Build history of the part. All positions in model axes, mm. Give positions to 0.01 mm unless a question says otherwise; leave off trailing zeros. Write each loop counter-clockwise with the first axis right and the second up, starting at its lowest first coordinate (ties: lowest second). Pieces come first, ordered by that corner, then holes. Notation, with made-up numbers: (-9, 82.5) -> (42, 82.5) arc R30 cw to (42, 108.5) -> close; hole circle Ø1 at (53, -29). An arc over 180 degrees is marked (long way). One line per question, with ' | ' between items. Start each with the question number.
(1) Drill centre lines: probe 1 along X at (y, z) = (-13, 20.5); probe 2 along Y at (x, z) = (-570, 12); probe 3 along Y at (x, z) = (710, 29). Where is each one in solid material? Low to high. Write a range as from..to.
(2) Band-saw the part on A-A, the plane x = -640. Give the cut face in (y, z).
(3) Pin check, flat tips, straight feed: P1, Ø6, axis at y = 208.5, z = 70, coming from the +X side; P2, Ø12, axis at x = 558, z = -15.5, coming from the -Y side; P3, Ø15, axis at x = -675.5, z = 18, coming from the +Y side. Stop position of each tip, or through.
(4) Band-saw the part on B-B, the plane x = 265.5. Give the cut face in (y, z).
from build123d import *

# Parameters (mm, degrees)
SKETCH1_W                = 200
SKETCH1_H                = 40
SKETCH1_R                = 5
SKETCH1_R_2              = 15
BOSS_EXTRUDE2_DEPTH      = 50
BOSS_EXTRUDE2_2_DEPTH    = 50
SKETCH2_R                = 7.5
BOSS_EXTRUDE4_DEPTH      = 40
BOSS_EXTRUDE5_DEPTH      = 250
BOSS_EXTRUDE5_DEPTH_BACK = 40
SKETCH3_R                = 7.5
SKETCH4_W                = 50
SKETCH4_H                = 100
BOSS_EXTRUDE6_DEPTH      = 50
SKETCH5_R                = 15
CUT_EXTRUDE1_DEPTH       = 1180
SKETCH6_W                = 50
SKETCH6_H                = 25
BOSS_EXTRUDE8_DEPTH      = 50
SKETCH7_R                = 5
BOSS_EXTRUDE9_DEPTH      = 1180
FILLET1_R                = 10


with BuildPart() as part:
    # Sketch1 → Boss-Extrude2 (new body)
    with BuildSketch(Plane.XY):
        with Locations((-640, -58.42888126)):
            Rectangle(SKETCH1_W, SKETCH1_H)
        with Locations((-710, -58.42888126)):
            Circle(SKETCH1_R, mode=Mode.SUBTRACT)
        with Locations((-570, -58.42888126)):
            Circle(SKETCH1_R, mode=Mode.SUBTRACT)
        with Locations((-640, -58.42888126)):
            Circle(SKETCH1_R_2, mode=Mode.SUBTRACT)
    extrude(amount=BOSS_EXTRUDE2_DEPTH)



with BuildPart() as body_2:
    # Sketch1 → Boss-Extrude2 2 (new body)
    with BuildSketch(Plane.XY):
        Polygon((580, -38.42888126), (540, -38.42888126), (540, -78.42888126), (740, -78.42888126), (740, -38.42888126), align=None)
        with Locations((570, -58.42888126)):
            Circle(SKETCH1_R, mode=Mode.SUBTRACT)
        with Locations((640, -58.42888126)):
            Circle(SKETCH1_R_2, mode=Mode.SUBTRACT)
        with Locations((710, -58.42888126)):
            Circle(SKETCH1_R, mode=Mode.SUBTRACT)
    extrude(amount=BOSS_EXTRUDE2_2_DEPTH)


with BuildPart() as part_1:
    add(part.part)

    add(body_2.part)  # Boss-Extrude4 merges body 2
    # Sketch2 → Boss-Extrude4 (add)
    # profile 1 of 2: a face of its own
    with BuildSketch(Plane(origin=(0, -38.42888126, 0), x_dir=(1, 0, 0), z_dir=(0, 1, 0))):
        Polygon((540, -25), (540, -75), (590, -75), (590, -25), (590, 25), (540, 25), align=None)
        with Locations(Location((566.239219394, 12.5, 0), (0, 0, 180))):
            Circle(SKETCH2_R, mode=Mode.SUBTRACT)
        with Locations(Location((566.239219394, -62.5, 0), (0, 0, 180))):
            Circle(SKETCH2_R, mode=Mode.SUBTRACT)
    # profile 2 of 2: a face of its own
    with BuildSketch(Plane(origin=(0, -38.42888126, 0), x_dir=(1, 0, 0), z_dir=(0, 1, 0))):
        Polygon((-590, -25), (-590, 25), (-540, 25), (-540, -25), (-540, -75), (-590, -75), align=None)
        with Locations(Location((-566.239219394, -62.5, 0), (0, 0, 180))):
            Circle(SKETCH2_R, mode=Mode.SUBTRACT)
        with Locations(Location((-566.239219394, 12.5, 0), (0, 0, 180))):
            Circle(SKETCH2_R, mode=Mode.SUBTRACT)
    extrude(amount=BOSS_EXTRUDE4_DEPTH)

    # Sketch3 → Boss-Extrude5 (add, two sides: drawn at the far end of the back side and taken through both)
    with BuildSketch(Plane(origin=(0, 0, 0), x_dir=(1, 0, 0), z_dir=(0, 1, 0)).offset(-BOSS_EXTRUDE5_DEPTH_BACK)):
        with Locations(Location((-566.239219394, 12.5, 0), (0, 0, 270))):
            Circle(SKETCH3_R)
        with Locations(Location((-566.239219394, -62.5, 0), (0, 0, 270))):
            Circle(SKETCH3_R)
        with Locations(Location((566.239219394, 12.5, 0), (0, 0, 270))):
            Circle(SKETCH3_R)
        with Locations(Location((566.239219394, -62.5, 0), (0, 0, 270))):
            Circle(SKETCH3_R)
    extrude(amount=BOSS_EXTRUDE5_DEPTH + BOSS_EXTRUDE5_DEPTH_BACK)

    # Sketch4 → Boss-Extrude6 (add)
    with BuildSketch(Plane(origin=(0, 250, 0), x_dir=(1, 0, 0), z_dir=(0, 1, 0))):
        with Locations((565, -25)):
            Rectangle(SKETCH4_W, SKETCH4_H)
        with Locations((-565, -25)):
            Rectangle(SKETCH4_W, SKETCH4_H)
    extrude(amount=-BOSS_EXTRUDE6_DEPTH)

    # Sketch5 → Cut-Extrude1 (cut)
    with BuildSketch(Plane.ZY.offset(590)):
        with Locations((25, 225)):
            Circle(SKETCH5_R)
    extrude(amount=-CUT_EXTRUDE1_DEPTH, mode=Mode.SUBTRACT)

    # Sketch6 → Boss-Extrude8 (add)
    with BuildSketch(Plane(origin=(0, 250, 0), x_dir=(1, 0, 0), z_dir=(0, 1, 0))):
        with Locations((565, -87.5)):
            Rectangle(SKETCH6_W, SKETCH6_H)
        with Locations((565, 37.5)):
            Rectangle(SKETCH6_W, SKETCH6_H)
        with Locations((-565, -87.5)):
            Rectangle(SKETCH6_W, SKETCH6_H)
        with Locations((-565, 37.5)):
            Rectangle(SKETCH6_W, SKETCH6_H)
    extrude(amount=-BOSS_EXTRUDE8_DEPTH)

    # Sketch7 → Boss-Extrude9 (add)
    with BuildSketch(Plane.ZY.offset(590)):
        with Locations(Location((87.5, 225, 0), (0, 0, 180))):
            Circle(SKETCH7_R)
        with Locations(Location((-37.5, 225, 0), (0, 0, 180))):
            Circle(SKETCH7_R)
    extrude(amount=-BOSS_EXTRUDE9_DEPTH)

    # Fillet1
    # the kernel refuses this fillet: 10 mm, written as the material it adds along each edge
    with BuildSketch(Plane(origin=(540, -38.42888126, 50), x_dir=(0, -1, 0), z_dir=(1, 0, 0)), Plane(origin=(590, -38.42888126, 0), x_dir=(0, -1, 0), z_dir=(-1, 0, 0)), Plane(origin=(-590, -38.42888126, 0), x_dir=(0, 0, -1), z_dir=(1, 0, 0))) as fillet1_piece_1:
        with BuildLine():
            CenterArc((FILLET1_R, -FILLET1_R), FILLET1_R, 90, 90)
            Line((0, -FILLET1_R), (0, 0))
            Line((0, 0), (FILLET1_R, 0))
        make_face()
    extrude(amount=50)
    with BuildSketch(Plane(origin=(-590, -38.42888126, 50), x_dir=(0, 0, 1), z_dir=(1, 0, 0))) as fillet1_piece_2:
        with BuildLine():
            CenterArc((FILLET1_R, FILLET1_R), FILLET1_R, 180, 90)
            Line((0, FILLET1_R), (0, 0))
            Line((0, 0), (FILLET1_R, 0))
        make_face()
    extrude(amount=50)


solid = part_1.part
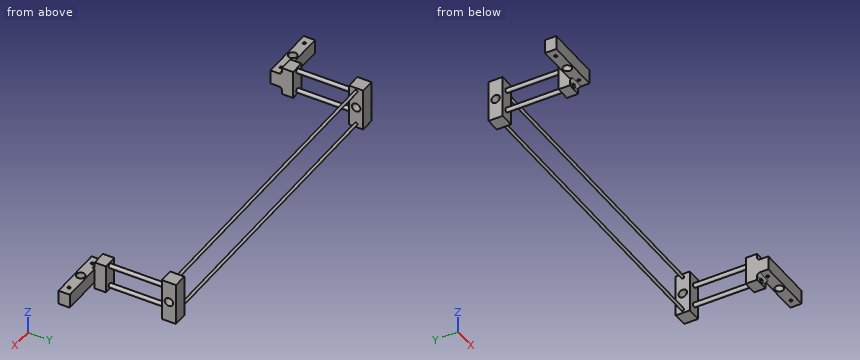
Results:
1) probe 1: x = -590..-540, 540..590 | probe 2: y = -78.43..-63.43, -53.43..1.57, 200..217.52, 232.48..250 | probe 3: y = -78.43..-63.43, -53.43..-38.43
2) outline: (-78.43, 0) -> (-73.43, 0) -> (-73.43, 50) -> (-78.43, 50) -> close; (-43.43, 0) -> (-38.43, 0) -> (-38.43, 50) -> (-43.43, 50) -> close
3) P1: stops at x = 590 | P2: stops at y = -40 | P3: stops at y = -38.43
4) outline: circle Ø10 at (225, -37.5); circle Ø10 at (225, 87.5)
